Part model, mm, in its own coordinate system. Coordinates: 2 decimals unless noted, no trailing zeros. Loops run counter-clockwise (first coordinate to the right, second up) from the corner with the lowest first, then second, coordinate; pieces in that order, holes last. Notation, with made-up numbers: M 32,61.25 L 79,61.25 A22 cw 79,73.25 Z; hole C 50,21 d5. An arc over 180 degrees is marked long. Answer as a JSON object with one key per item and string values. Group by question number.
1. Saw through at B-B on x = -30.5. Write the cut outline in (y, z), then the cut area to 3 significant figures.
2. Drop flat-ended pins along their axis: pin 1 Ø10 at (x, y) = (-28, 15) entering from -Z; pin 2 Ø9 at (x, y) = (2, -2) entering from +Z. Give the stop position or say it passes through.
3. Saw through at A-A on z = 94.5. Write the cut outline in (x, y), then the cut area to 4 significant figures.
4. Drill centre lines: L1, parallel to Y at x = -21, z = 79; L2, parallel to X at y = 0.5, z = 40; L3, parallel to Z at x = -22, y = 0.5. Where is each one in solid material? Low to high.
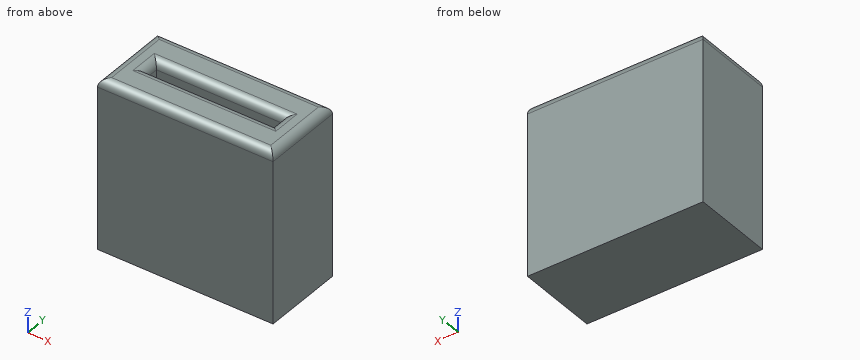
Autodesk Fusion 360 part; units mm, degrees
sketch "Sketch1" plane through (0, 0, 0) normal (0, 0, 1) x (1, 0, 0)
  line L0 (53.75, -25) -> (-53.75, -25)
  line L1 (-53.75, -25) -> (-53.75, 25)
  line L2 (-53.75, 25) -> (53.75, 25)
  line L3 (53.75, 25) -> (53.75, -25)
  line L4 (53.75, -25) -> (-53.75, 25) construction
  line L5 (-53.75, -25) -> (53.75, 25) construction
  dimension "d4" = 107.5
  dimension "d5" = 50
extrude "Extrude1" add sketch "Sketch1" along normal blind 104
sketch "Sketch2" plane through (0, 0, 104) normal (0, 0, 1) x (-1, 0, 0)
  line L0 (-53.75, -25) -> (53.75, -25)
  line L1 (53.75, -25) -> (53.75, 25)
  line L2 (53.75, 25) -> (-53.75, 25)
  line L3 (-53.75, 25) -> (-53.75, -25)
  line L4 (-38.75, 4) -> (38.75, 4)
  line L5 (38.75, 4) -> (38.75, -4)
  line L6 (38.75, -4) -> (-38.75, -4)
  line L7 (-38.75, -4) -> (-38.75, 4)
  line L8 (-38.75, 4) -> (38.75, -4) construction
  line L9 (38.75, 4) -> (-38.75, -4) construction
  dimension "d8" = 77.5
  dimension "d9" = 8
extrude "Extrude2" cut sketch "Sketch2" against normal blind 94 contours L4 L5 L6 L7
fillet "Fillet1" radius 5 1 faces at (12.9167, -18, 104)
equation "bredde = 77.5 mm"
equation "tykkelse = 8 mm"
equation "d4 = bredde + 30 mm"
equation "d8 = bredde"
equation "d9 = tykkelse"
Outcome:
{
 "1": {"outline": "M -25,0 L 25,0 L 25,99 A5 ccw 20,104 L 9,104 A5 ccw 4,99 L 4,10 L -4,10 L -4,99 A5 ccw -9,104 L -20,104 A5 ccw -25,99 Z", "area": "4,430 mm²"},
 "2": {"pin 1": "stops at z = 0", "pin 2": "stops at z = 103.33"},
 "3": {"outline": "M -53.75,-25 L 53.75,-25 L 53.75,25 L -53.75,25 Z; hole M -38.75,-4 L 38.75,-4 L 38.75,4 L -38.75,4 Z", "area": "4,755 mm²"},
 "4": {"L1": "y = -25 to -4, 4 to 25", "L2": "x = -53.75 to -38.75, 38.75 to 53.75", "L3": "z = 0 to 10"}
}
